Model file for the job. Use its own axes, mm. A direction names the side the tool comes from. Round coordinates to 2 decimals unless told otherwise and drop trailing zeros. Loops run counter-clockwise (first coordinate to the right, second up) from the corner with the lowest first, then second, coordinate; pieces in that order, holes last. Notation, with made-up numbers: (85, 66) -> (113, 66) arc R24 ccw to (113, 79) -> close; hole circle Ø3 at (84.5, 18). An arc over 180 degrees is marked (long way). Use a Markdown table: item, result.
from build123d import *

# Parameters (mm, degrees)
SKETCH1_R           = 62.5
BOSS_EXTRUDE1_DEPTH = 21
SKETCH2_R           = 32
SKETCH2_R_2         = 6
CUT_EXTRUDE1_DEPTH  = 16
SKETCH3_R           = 6
SKETCH3_R_2         = 4
CUT_EXTRUDE2_DEPTH  = 14
SKETCH4_R           = 4
CUT_EXTRUDE3_DEPTH  = 7.5
CUT_EXTRUDE4_START  = -5
CUT_EXTRUDE4_DEPTH  = 5
CUT_EXTRUDE5_START  = -5
CUT_EXTRUDE5_DEPTH  = 5
CUT_EXTRUDE6_START  = -5
CUT_EXTRUDE6_DEPTH  = 5


# Read off the part's stored shape, not the designer's step: Cut-Extrude6
with BuildPart() as part:
    # Sketch1 → Boss-Extrude1 (new body)
    with BuildSketch(Plane(origin=(0, 0, 0), x_dir=(1, 0, 0), z_dir=(0, 1, 0))):
        with Locations(Location((0, 0, 0), (0, 0, 90))):
            Circle(SKETCH1_R)
    extrude(amount=BOSS_EXTRUDE1_DEPTH)

    # Sketch2 → Cut-Extrude1 (cut)
    with BuildSketch(Plane(origin=(0, 21, 0), x_dir=(1, 0, 0), z_dir=(0, 1, 0))):
        with Locations(Location((0, 0, 0), (0, 0, 270))):
            Circle(SKETCH2_R)
        with Locations(Location((0, 0, 0), (0, 0, 270))):
            Circle(SKETCH2_R_2, mode=Mode.SUBTRACT)
    extrude(amount=-CUT_EXTRUDE1_DEPTH, mode=Mode.SUBTRACT)

    # Sketch3 → Cut-Extrude2 (cut)
    with BuildSketch(Plane(origin=(0, 21, 0), x_dir=(1, 0, 0), z_dir=(0, 1, 0))):
        with Locations(Location((0, 0, 0), (0, 0, 270))):
            Circle(SKETCH3_R)
        with Locations(Location((0, 0, 0), (0, 0, 270))):
            Circle(SKETCH3_R_2, mode=Mode.SUBTRACT)
    extrude(amount=-CUT_EXTRUDE2_DEPTH, mode=Mode.SUBTRACT)

    # Sketch4 → Cut-Extrude3 (cut)
    with BuildSketch(Plane(origin=(0, 21, 0), x_dir=(1, 0, 0), z_dir=(0, 1, 0))):
        with Locations(Location((0, 0, 0), (0, 0, 270))):
            Circle(SKETCH4_R)
    extrude(amount=-CUT_EXTRUDE3_DEPTH, mode=Mode.SUBTRACT)

    # Sketch5 → Cut-Extrude4 (cut)
    with BuildSketch(Plane(origin=(0, 21, 0), x_dir=(1, 0, 0), z_dir=(0, 1, 0)).offset(CUT_EXTRUDE4_START)):
        with BuildLine():
            Line((2.05, 62.466370953), (2.05, -62.466370953))
            ThreePointArc((2.05, -62.466370953), (0, -62.5), (-2.05, -62.466370953))
            Line((-2.05, -62.466370953), (-2.05, 62.466370953))
            ThreePointArc((-2.05, 62.466370953), (0, 62.5), (2.05, 62.466370953))
        make_face()
    extrude(amount=CUT_EXTRUDE4_DEPTH, mode=Mode.SUBTRACT)

    # Sketch6 → Cut-Extrude5 (cut)
    with BuildSketch(Plane(origin=(0, 21, 0), x_dir=(1, 0, 0), z_dir=(0, 1, 0)).offset(CUT_EXTRUDE5_START)):
        with BuildLine():
            Line((-48.35, -39.60463988), (48.35, -39.60463988))
            ThreePointArc((48.35, -39.60463988), (49.936833573, -37.584074456), (51.439284598, -35.5))
            Line((51.439284598, -35.5), (-51.439284598, -35.5))
            ThreePointArc((-51.439284598, -35.5), (-49.936833573, -37.584074456), (-48.35, -39.60463988))
        make_face()
    extrude(amount=CUT_EXTRUDE5_DEPTH, mode=Mode.SUBTRACT)

    # Cut-Extrude6 outline → Cut-Extrude6 (cut)
    with BuildSketch(Plane(origin=(0, 21, 0), x_dir=(1, 0, 0), z_dir=(0, 1, 0)).offset(CUT_EXTRUDE6_START)):
        with BuildLine():
            Line((6.37014237, -42.848279801), (6.37014237, -46.848279801))
            Line((6.37014237, -46.848279801), (41.37014237, -46.848279801))
            ThreePointArc((41.37014237, -46.848279801), (43.481229311, -44.895798217), (45.500273824, -42.848279801))
            Line((45.500273824, -42.848279801), (6.37014237, -42.848279801))
        make_face()
    extrude(amount=CUT_EXTRUDE6_DEPTH, mode=Mode.SUBTRACT)


solid = part.part
Q1. Band-saw the part on C-C, the plane z = 0. Give the cut face in (x, y), plus the area to 3 significant figures.
Results list:
| item | result |
|---|---|
| outline | (-62.5, 0) -> (62.5, 0) -> (62.5, 21) -> (32, 21) -> (32, 5) -> (6, 5) -> (6, 7) -> (4, 7) -> (4, 13.5) -> (-4, 13.5) -> (-4, 7) -> (-6, 7) -> (-6, 5) -> (-32, 5) -> (-32, 21) -> (-62.5, 21) -> close |
| area | 1,680 mm² |
Q2. Band-saw the part on B-B, the plane x = 0. Give the cut face in (y, z).
Results list:
| item | result |
|---|---|
| outline | (0, -62.5) -> (16, -62.5) -> (16, -32) -> (5, -32) -> (5, -6) -> (7, -6) -> (7, -4) -> (13.5, -4) -> (13.5, 4) -> (7, 4) -> (7, 6) -> (5, 6) -> (5, 32) -> (16, 32) -> (16, 62.5) -> (0, 62.5) -> close |
Q3. Flat gauge pins, fed straight in: pin 1 (1.8 mm diameter, centred on y = 19.5, z = 34, fed in from -X); pin 2 (1.5 mm diameter, centred on x = 32, y = 19, fed in from -Z); pin 3 (4 mm diameter, centred on y = 5, z = 17, fed in from -X). Where does each tip first touch, or does it go through?
Results list:
| item | result |
|---|---|
| pin 1 | stops at x = -53.02 |
| pin 2 | stops at z = -54.13 |
| pin 3 | stops at x = -60.67 |
Q4. Drill centre lines: L1, parallel to X at y = 9.75, z = 0; L2, parallel to X at y = 15, z = 0; L3, parallel to Z at x = 3.5, y = 17. Where is each one in solid material? Low to high. Write a range as from..to.
Results list:
| item | result |
|---|---|
| L1 | x = -62.5..-32, -4..4, 32..62.5 |
| L2 | x = -62.5..-32, 32..62.5 |
| L3 | z = -62.4..-31.81, 31.81..35.5, 39.6..62.4 |
Q5. Pull direction X, two halves, no side cores. Call faces 5 (the face through (-18.773, 10.353, -59.614)), 6 (the face through (0, 16, 40)), 7 (the face through (-20, 21, 49)): released by +X, released by -X, zero draft, split by the parting line, or undercut.
Results list:
| item | result |
|---|---|
| face 5 | split by the parting line |
| face 6 | undercut |
| face 7 | zero draft |
Q6. Tool access for faces 1 (the face through (25, 18, 39.605)), 2 (the face through (-3.905, 10.296, -0.867)), 3 (the face through (26, 18, 42.848)), 4 (the face through (2.05, 18, 34)): list every direction of +Z, -Z, +X, -X, +Y, -Y with a clear straight run to the whole face (end or side of a thin tool).
Results list:
| item | result |
|---|---|
| face 1 | +X, -X, +Y |
| face 2 | +Y |
| face 3 | +X, +Y |
| face 4 | +Z, -Z, +Y |
Q7. Band-saw the part on D-D, the plane y = 3.25. Give the cut face in (x, z), plus the area to 3 significant figures.
Results list:
| item | result |
|---|---|
| outline | circle Ø125 at (0, 0) |
| area | 12,300 mm² |
Q8. Band-saw the part on A-A, the plane y = 10.25. Give the cut face in (x, z).
Results list:
| item | result |
|---|---|
| outline | circle Ø125 at (0, 0); circle Ø8 at (0, 0); hole circle Ø64 at (0, 0) |
